```python
from build123d import *

# Parameters (mm, degrees)
SKETCH1_W           = 12
SKETCH1_H           = 15
SKETCH1_R           = 1.5
BOSS_EXTRUDE1_DEPTH = 3
CUT_EXTRUDE1_REACH  = 12.062


with BuildPart() as part:
    # Sketch1 → Boss-Extrude1 (new body)
    with BuildSketch(Plane.XY):
        Rectangle(SKETCH1_W, SKETCH1_H)
        with Locations((-3, -4.5)):
            Circle(SKETCH1_R, mode=Mode.SUBTRACT)
        with Locations((3, -4.5)):
            Circle(SKETCH1_R, mode=Mode.SUBTRACT)
    extrude(amount=BOSS_EXTRUDE1_DEPTH)

    # Sketch2 → Cut-Extrude1 (cut, up to next)
    with BuildSketch(Plane.XY.offset(3), mode=Mode.PRIVATE) as cut_extrude1_sk1:
        with BuildLine():
            Line((-3, 7.5), (3, 7.5))
            Line((3, 7.5), (3, 2.5))
            ThreePointArc((3, 2.5), (0, -0.5), (-3, 2.5))
            Line((-3, 2.5), (-3, 7.5))
        make_face()
    cut_extrude1_tool1 = extrude(cut_extrude1_sk1.sketch, amount=-CUT_EXTRUDE1_REACH, mode=Mode.PRIVATE) & part.part
    add(cut_extrude1_tool1.solids().sort_by_distance((0, 3.791429, 3))[0], mode=Mode.SUBTRACT)


solid = part.part
```
For this review, take the finished solid that the model builds, in its own axes (mm). A direction names the side the tool comes from. Coordinates: 2 decimals unless noted, no trailing zeros. Order: outer loops, then holes, each group sorted by start corner. A loop starts at its lowest first (then second) coordinate and runs counter-clockwise, first axis right, second up. Notation, with made-up numbers: (-28.5, -35) -> (30.5, -35) arc R24 ccw to (30.5, -20) -> close; hole circle Ø2 at (25.5, -30.5). An arc over 180 degrees is marked (long way). Use CSV: the item, a comma, the result in double quotes. Start each with the question number.
Item 1: We need section C-C, the plane y = 2. Give the boundary of the cut face in (x, z), then the cut area to 3 significant figures.
Item 2: For faces 1 (the face through (3, 5, 2)), 2 (the face through (6, 0, 1)), list the 3-axis set-ups (+Z, -Z, +X, -X, +Y, -Y) from which the entire face can be reached by the end or side of a thin tool; tool diameter is ignored.
Item 3: Draft analysis for pull direction X (two halves, no side actions). For faces 3 (the face through (-5, 7.5, 1)), 4 (the face through (-1.57, -4.05, 1.48)), 5 (the face through (-6, 0, 1)), state which applies: pulls with the +X half, pulls with the -X half, needs draft (parallel to the pull), parting line crosses it, or undercut.
Item 4: We need section B-B, the plane x = -3.75. Give the boundary of the cut face in (y, z).
Item 5: Wall thickness on probe 1 along X at (y, z) = (4.5, 1.7); probe 2 along X at (y, z) = (-5.5, 1.5); probe 3 along X at (y, z) = (0, 2.15): over which ranges is each line inside the solid? List them lowest first.
Item 6: We need section D-D, the plane z = 0.35. Give the boundary of the cut face in (x, y).
Item 7: We need section A-A, the plane y = -4.5. Give the boundary of the cut face in (x, z), then the cut area to 3 significant figures.
Item 8: Insertion check: pin 1 (1 mm diameter, centred on x = 0, z = 1, fed in from +Y). The pin has a flat end and moves straight along its axis. Give the tip position at first contact, or say it passes through.
Derived:
1,outline,"(-6, 0) -> (-2.96, 0) -> (-2.96, 3) -> (-6, 3) -> close; (2.96, 0) -> (6, 0) -> (6, 3) -> (2.96, 3) -> close"
1,area,"18.3 mm^2"
2,face 1,"+Z, -Z, +Y"
2,face 2,"+Z, -Z, +X, +Y, -Y"
3,face 3,"needs draft"
3,face 4,"undercut"
3,face 5,"pulls with the -X half"
4,outline,"(-7.5, 0) -> (-5.8, 0) -> (-5.8, 3) -> (-7.5, 3) -> close; (-3.2, 0) -> (7.5, 0) -> (7.5, 3) -> (-3.2, 3) -> close"
5,probe 1,"x = -6 to -3, 3 to 6"
5,probe 2,"x = -6 to -4.12, -1.88 to 1.88, 4.12 to 6"
5,probe 3,"x = -6 to -1.66, 1.66 to 6"
6,outline,"(-6, -7.5) -> (6, -7.5) -> (6, 7.5) -> (3, 7.5) -> (3, 2.5) arc R3 cw to (-3, 2.5) -> (-3, 7.5) -> (-6, 7.5) -> close; hole circle Ø3 at (-3, -4.5); hole circle Ø3 at (3, -4.5)"
7,outline,"(-6, 0) -> (-4.5, 0) -> (-4.5, 3) -> (-6, 3) -> close; (-1.5, 0) -> (1.5, 0) -> (1.5, 3) -> (-1.5, 3) -> close; (4.5, 0) -> (6, 0) -> (6, 3) -> (4.5, 3) -> close"
7,area,"18.0 mm^2"
8,pin 1,"stops at y = -0.46"
